Check sheet for the modelled part. Datum: model origin and axes. Units: mm. A direction names the side the tool comes from. Coordinates: 2 decimals unless noted, no trailing zeros. Write each loop counter-clockwise with the first axis right and the second up, starting at its lowest first coordinate (ties: lowest second). Pieces come first, ordered by that corner, then holes. Notation, with made-up numbers: (52, 47) - (98, 47) arc R27 cw to (98, 81) - close; hole circle Ø10 at (-22.75, 26). An arc over 180 degrees is marked (long way). Write each question's results on one line, items separated by ' | '.
from build123d import *

# Parameters (mm, degrees)
SKETCH1_R           = 3.175
BOSS_EXTRUDE2_DEPTH = 46.99
BOSS_EXTRUDE3_DEPTH = 10.16
SKETCH3_R           = 3.175
SKETCH3_R_2         = 1.778
CUT_EXTRUDE1_DEPTH  = 19.05
SKETCH6_R           = 3.175
BOSS_EXTRUDE5_DEPTH = 49.022
CUT_EXTRUDE5_DEPTH  = 38.1
SKETCH9_R           = 0.866025404
CUT_EXTRUDE7_DEPTH  = 46.99
SKETCH10_R          = 0.8001
CUT_EXTRUDE8_DEPTH  = 5.334
CUT_EXTRUDE9_START  = 0.762
SKETCH11_R          = 3.175
SKETCH11_R_2        = 2.667
CUT_EXTRUDE9_DEPTH  = 0.762
CUT_EXTRUDE10_START = 0.762
SKETCH12_R          = 3.175
SKETCH12_R_2        = 2.667
CUT_EXTRUDE10_DEPTH = 0.762
CUT_EXTRUDE12_START = 0.762
SKETCH13_R          = 3.175
SKETCH13_R_2        = 2.667
CUT_EXTRUDE12_DEPTH = 0.762


with BuildPart() as part:
    # Sketch1 → Boss-Extrude2 (new body)
    with BuildSketch(Plane(origin=(0, 0, 0), x_dir=(0, 0, -1), z_dir=(1, 0, 0))):
        Circle(SKETCH1_R)
    extrude(amount=BOSS_EXTRUDE2_DEPTH)

    # Sketch2 → Boss-Extrude3 (add)
    with BuildSketch(Plane(origin=(46.99, 0, 0), x_dir=(0, 0, -1), z_dir=(1, 0, 0))):
        Polygon((-5.499261314, 3.175), (-5.499261314, -3.175), (0, -6.35), (5.499261314, -3.175), (5.499261314, 3.175), (0, 6.35), align=None)
    extrude(amount=BOSS_EXTRUDE3_DEPTH)

    # Sketch3 → Cut-Extrude1 (cut)
    with BuildSketch(Plane.ZY):
        Circle(SKETCH3_R)
        Circle(SKETCH3_R_2, mode=Mode.SUBTRACT)
    extrude(amount=-CUT_EXTRUDE1_DEPTH, mode=Mode.SUBTRACT)

    # Sketch6 → Boss-Extrude5 (add)
    with BuildSketch(Plane.ZY):
        Circle(SKETCH6_R)
    extrude(amount=-BOSS_EXTRUDE5_DEPTH)

    # Sketch7 → Cut-Extrude5 (cut)
    with BuildSketch(Plane.ZY):
        Polygon((-0.489261374, 0.714579112), (-0.863474351, -0.066423223), (-0.374212977, -0.781002335), (0.489261374, -0.714579112), (0.863474351, 0.066423223), (0.374212977, 0.781002335), align=None)
    extrude(amount=-CUT_EXTRUDE5_DEPTH, mode=Mode.SUBTRACT)

    # Sketch9 → Cut-Extrude7 (cut)
    with BuildSketch(Plane.ZY):
        Circle(SKETCH9_R)
    extrude(amount=-CUT_EXTRUDE7_DEPTH, mode=Mode.SUBTRACT)

    # Sketch10 → Cut-Extrude8 (cut)
    with BuildSketch(Plane.XY.offset(5.499261314)):
        with Locations((3.81, 0)):
            Circle(SKETCH10_R)
    extrude(amount=-CUT_EXTRUDE8_DEPTH, mode=Mode.SUBTRACT)

    # Sketch11 → Cut-Extrude9 (cut)
    with BuildSketch(Plane.ZY.offset(-36.5125).offset(CUT_EXTRUDE9_START)):
        Circle(SKETCH11_R)
        with Locations(Location((0, 0, 0), (0, 0, 180))):
            Circle(SKETCH11_R_2, mode=Mode.SUBTRACT)
    extrude(amount=-CUT_EXTRUDE9_DEPTH, mode=Mode.SUBTRACT)

    # Sketch12 → Cut-Extrude10 (cut)
    with BuildSketch(Plane.ZY.offset(-15.875).offset(CUT_EXTRUDE10_START)):
        Circle(SKETCH12_R)
        with Locations(Location((0, 0, 0), (0, 0, 180))):
            Circle(SKETCH12_R_2, mode=Mode.SUBTRACT)
    extrude(amount=-CUT_EXTRUDE10_DEPTH, mode=Mode.SUBTRACT)

    # Sketch13 → Cut-Extrude12 (cut)
    with BuildSketch(Plane.ZY.offset(-22.987).offset(CUT_EXTRUDE12_START)):
        Circle(SKETCH13_R)
        with Locations(Location((0, 0, 0), (0, 0, 180))):
            Circle(SKETCH13_R_2, mode=Mode.SUBTRACT)
    extrude(amount=-CUT_EXTRUDE12_DEPTH, mode=Mode.SUBTRACT)


solid = part.part
1. Draft check along Z on faces 1 (the cylindrical face through (23.166, -0.845, -0.188)), 2 (the flat face through (52, 0, 5.499)), 3 (the flat face through (22.987, 2, -2)). Enter one of: pulls with the +Z half, pulls with the -Z half, needs draft (parallel to the pull), parting line crosses it, or undercut.
Values follow:
face 1: undercut | face 2: pulls with the +Z half | face 3: needs draft
2. Sectioned sample at A-A (x = 51.5). Record the cut outline in (y, z) (3 decimals).
Values follow:
outline: (-6.35, 0) - (-3.175, -5.499) - (3.175, -5.499) - (6.35, 0) - (3.175, 5.499) - (-3.175, 5.499) - close
3. Go/stop test with flat-tipped pins: pin 1 (2 mm diameter, centred on x = 16, y = -5, fed in from +Z); pin 2 (5 mm diameter, centred on y = -0.5, z = -0.5, fed in from -X); pin 3 (1 mm diameter, centred on x = 8, z = -0.5, fed in from +Y) (3 decimals); pin 4 (2 mm diameter, centred on x = 3.81, y = 0, fed in from +Z) (3 decimals). Record where each tip stops, or that it passes through.
Values follow:
pin 1: passes through | pin 2: stops at x = 0 | pin 3: stops at y = 3.175 | pin 4: stops at z = 3.175
4. Access from +Z, -Z, +X, -X, +Y, -Y to the whole of each face (thin tool, end or side, straight path). Record for faces 4 (the flat face through (51.999, 4.785, 2.711)), 5 (the flat face through (46.99, -3, 3)), 6 (the cylindrical face through (22.601, 2.366, -1.231)).
Values follow:
face 4: +Z, +X, -X, +Y | face 5: -X | face 6: none
5. Sectioned sample at C-C (x = 37). Record the cut outline in (y, z) (3 decimals), then the cut area to 3 significant figures.
Values follow:
outline: circle Ø6.35 at (0, 0); hole circle Ø1.732 at (0, 0) | area: 29.3 mm^2
6. Material ranges on L1, parallel to Y at x = 11, z = 0 (3 decimals); L2, parallel to X at y = -3.5, z = 4; L3, parallel to Y at x = 3.81, z = 1.9, recorded low to high. Write a range as [from, to].
Values follow:
L1: y = [-3.175, -0.866], [0.866, 3.175] | L2: x = [46.99, 57.15] | L3: y = [-2.54, -0.8], [0.8, 2.54]
